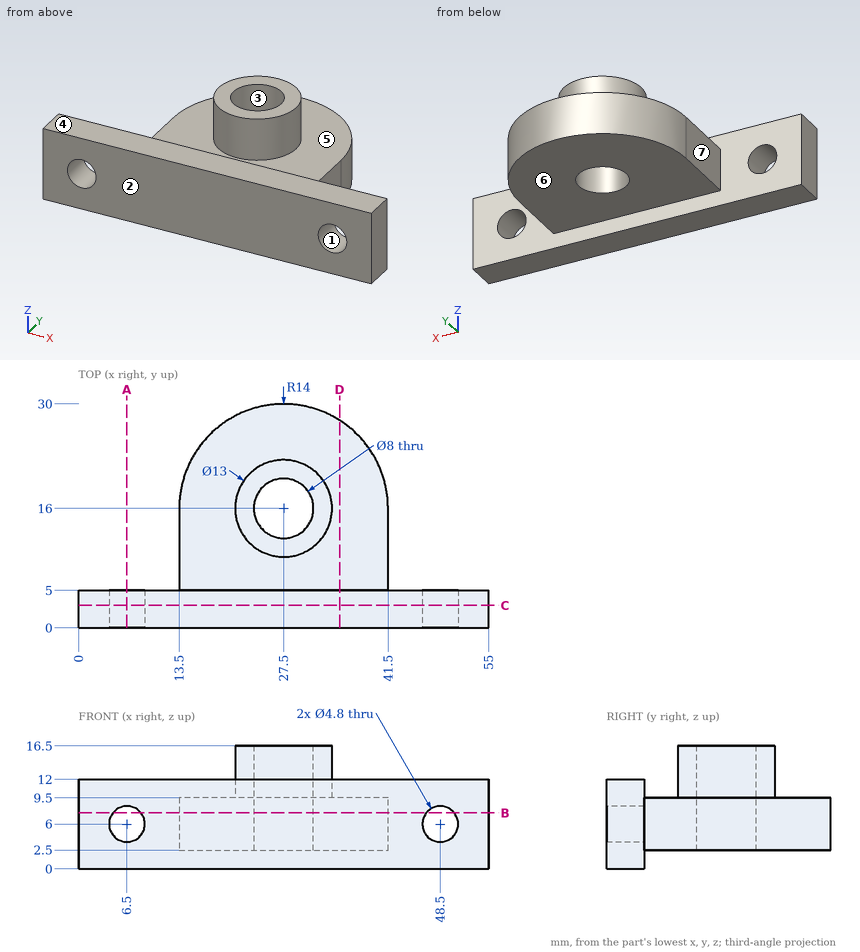
The figure shows three views and two pictorial views of one solid part (mm, origin at its lowest corner). Answer the questions. A direction names the side the tool comes from. Coordinates: 2 decimals unless noted, no trailing zeros. Loops run counter-clockwise (first coordinate to the right, second up) from the corner with the lowest first, then second, coordinate; pieces in that order, holes last.
(1) The part is cut by section D-D (x = 35). Determine the outline of the cut face in (y, z).
Solution:
outline: (0, 0) - (5, 0) - (5, 2.5) - (27.82, 2.5) - (27.82, 9.5) - (5, 9.5) - (5, 12) - (0, 12) - close
(2) Flat-ended cylindrical pins translate along their axes: pin 1 Ø1.5 at (y, z) = (21.5, 5.5) entering from +X; pin 2 Ø3 at (y, z) = (21, 9.5) entering from +X; pin 3 Ø6.5 at (x, y) = (27.5, 16) entering from -Z; pin 4 Ø5.5 at (y, z) = (12, 4.5) entering from +X. Find the tip coordinate at first contact, or state that the pin passes through.
Solution:
pin 1: stops at x = 40.67
pin 2: stops at x = 41.06
pin 3: passes through
pin 4: stops at x = 41.5
(3) The part is cut by section C-C (y = 3). Determine the outline of the cut face in (x, z).
Solution:
outline: (0, 0) - (55, 0) - (55, 12) - (0, 12) - close; hole circle Ø4.8 at (6.5, 6); hole circle Ø4.8 at (48.5, 6)
(4) The part is cut by section B-B (z = 7.5). Determine the outline of the cut face in (x, y), and give its area (3 significant figures).
Solution:
outline: (0, 0) - (4.63, 0) - (4.63, 5) - (0, 5) - close; (8.37, 0) - (46.63, 0) - (46.63, 5) - (41.5, 5) - (41.5, 16) arc R14 ccw to (13.5, 16) - (13.5, 5) - (8.37, 5) - close; (50.37, 0) - (55, 0) - (55, 5) - (50.37, 5) - close; hole circle Ø8 at (27.5, 16)
area: 803 mm2
(5) A tool of negligible diameter and unlimited length cuts with its end or side. For the marked faces 4, 5, 6 and 7, from which of +Z, -Z, +X, -X, +Y, -Y can it reach the whole face along a straight path? Write none if from no direction.
Solution:
face 4: +Z, +X, -X, -Y
face 5: +Z
face 6: -Z, +X, -X, +Y
face 7: +Z, -Z, -X, +Y
(6) The mould has two halves that part along Y. Classify the marked faces 1, 2 and 3: released by +Y, released by -Y, zero draft, split by the parting line, or undercut.
Solution:
face 1: zero draft
face 2: released by -Y
face 3: undercut
(7) The part is cut by section A-A (x = 6.5). Determine the outline of the cut face in (y, z), and give its area (3 significant figures).
Solution:
outline: (0, 0) - (5, 0) - (5, 3.6) - (0, 3.6) - close; (0, 8.4) - (5, 8.4) - (5, 12) - (0, 12) - close
area: 36.0 mm2
(8) Consider line 1 along X through (y, z) = (2.65, 6); line 2 along Y through (x, z) = (27.5, 13.5); line 3 along Z through (x, y) = (23, 28.5). Determine where each line is inside the solid, lowest interval first.
Solution:
line 1: x = 0 to 4.1, 8.9 to 46.1, 50.9 to 55
line 2: y = 9.5 to 12, 20 to 22.5
line 3: z = 2.5 to 9.5
